```python
from build123d import *

# Parameters (mm, degrees)
SKETCH1_W                      = 58.7
SKETCH1_H                      = 85.15
SKETCH1_W_2                    = 230
SKETCH1_H_2                    = 50
BOSS_EXTRUDE1_DEPTH            = 10
M5_CLEARANCE_HOLE1_D           = 5.5
M5_CLEARANCE_HOLE1_CSINK_D     = 5.55
M5_CLEARANCE_HOLE1_CSINK_ANGLE = 90
SKETCH5_W                      = 40
SKETCH5_H                      = 50
CUT_EXTRUDE1_DEPTH             = 5
FILLET1_R                      = 10


# Read off the part's stored shape, not the designer's step: M5 Clearance Hole2
with BuildPart() as part:
    # Sketch1 → Boss-Extrude1 (new body)
    with BuildSketch(Plane(origin=(0, 0, 0), x_dir=(1, 0, 0), z_dir=(0, 1, 0))):
        with Locations((0, 67.575)):
            Rectangle(SKETCH1_W, SKETCH1_H)
        Rectangle(SKETCH1_W_2, SKETCH1_H_2)
    extrude(amount=BOSS_EXTRUDE1_DEPTH)

    # M5 Clearance Hole1 (through all)
    with Locations(Plane(origin=(0, 10, 0), x_dir=(1, 0, 0), z_dir=(0, 1, 0))):
        with Locations((-21.85, 52), (21.85, 52)):
            CounterSinkHole(M5_CLEARANCE_HOLE1_D / 2, M5_CLEARANCE_HOLE1_CSINK_D / 2, counter_sink_angle=M5_CLEARANCE_HOLE1_CSINK_ANGLE)

    # Sketch5 → Cut-Extrude1 (cut)
    with BuildSketch(Plane.XZ):
        with Locations((-95, 0)):
            Rectangle(SKETCH5_W, SKETCH5_H)
        with Locations((95, 0)):
            Rectangle(SKETCH5_W, SKETCH5_H)
    extrude(amount=-CUT_EXTRUDE1_DEPTH, mode=Mode.SUBTRACT)

    # M5 Clearance Hole2 outline → M5 Clearance Hole2 (revolve, cut)
    with BuildSketch(Plane(origin=(-85, 0, -15), x_dir=(1, 0, 0), z_dir=(0, 0, 1))):
        Polygon((2.75, 5.025), (2.75, 10), (0, 10), (0, 5), (2.775, 5), align=None)
    revolve(axis=Axis((-85, 0, -15), (0, 1, 0)), mode=Mode.SUBTRACT)

    # M5 Clearance Hole2 2 outline → M5 Clearance Hole2 2 (revolve, cut)
    with BuildSketch(Plane(origin=(-85, 0, 15), x_dir=(1, 0, 0), z_dir=(0, 0, 1))):
        Polygon((2.75, 5.025), (2.75, 10), (0, 10), (0, 5), (2.775, 5), align=None)
    revolve(axis=Axis((-85, 0, 15), (0, 1, 0)), mode=Mode.SUBTRACT)

    # M5 Clearance Hole2 3 outline → M5 Clearance Hole2 3 (revolve, cut)
    with BuildSketch(Plane(origin=(-105, 0, -15), x_dir=(1, 0, 0), z_dir=(0, 0, 1))):
        Polygon((2.75, 5.025), (2.75, 10), (0, 10), (0, 5), (2.775, 5), align=None)
    revolve(axis=Axis((-105, 0, -15), (0, 1, 0)), mode=Mode.SUBTRACT)

    # M5 Clearance Hole2 4 outline → M5 Clearance Hole2 4 (revolve, cut)
    with BuildSketch(Plane(origin=(-105, 0, 15), x_dir=(1, 0, 0), z_dir=(0, 0, 1))):
        Polygon((2.75, 5.025), (2.75, 10), (0, 10), (0, 5), (2.775, 5), align=None)
    revolve(axis=Axis((-105, 0, 15), (0, 1, 0)), mode=Mode.SUBTRACT)

    # M5 Clearance Hole2 5 outline → M5 Clearance Hole2 5 (revolve, cut)
    with BuildSketch(Plane(origin=(105, 0, -15), x_dir=(1, 0, 0), z_dir=(0, 0, 1))):
        Polygon((2.75, 5.025), (2.75, 10), (0, 10), (0, 5), (2.775, 5), align=None)
    revolve(axis=Axis((105, 0, -15), (0, 1, 0)), mode=Mode.SUBTRACT)

    # M5 Clearance Hole2 6 outline → M5 Clearance Hole2 6 (revolve, cut)
    with BuildSketch(Plane(origin=(105, 0, 15), x_dir=(1, 0, 0), z_dir=(0, 0, 1))):
        Polygon((2.75, 5.025), (2.75, 10), (0, 10), (0, 5), (2.775, 5), align=None)
    revolve(axis=Axis((105, 0, 15), (0, 1, 0)), mode=Mode.SUBTRACT)

    # M5 Clearance Hole2 7 outline → M5 Clearance Hole2 7 (revolve, cut)
    with BuildSketch(Plane(origin=(85, 0, -15), x_dir=(1, 0, 0), z_dir=(0, 0, 1))):
        Polygon((2.75, 5.025), (2.75, 10), (0, 10), (0, 5), (2.775, 5), align=None)
    revolve(axis=Axis((85, 0, -15), (0, 1, 0)), mode=Mode.SUBTRACT)

    # M5 Clearance Hole2 8 outline → M5 Clearance Hole2 8 (revolve, cut)
    with BuildSketch(Plane(origin=(85, 0, 15), x_dir=(1, 0, 0), z_dir=(0, 0, 1))):
        Polygon((2.75, 5.025), (2.75, 10), (0, 10), (0, 5), (2.775, 5), align=None)
    revolve(axis=Axis((85, 0, 15), (0, 1, 0)), mode=Mode.SUBTRACT)

    # Fillet1
    fillet1_edges = [part.edges().sort_by_distance(p)[0] for p in [
        (-29.35, 5, -110.15),
        (29.35, 5, -110.15),
        (29.35, 5, -25),
        (-29.35, 5, -25),
    ]]
    fillet(fillet1_edges, radius=FILLET1_R)


solid = part.part
```
Part model, mm, in its own coordinate system. A direction names the side the tool comes from. Give positions to 0.01 mm unless a question says otherwise; leave off trailing zeros. Loops run counter-clockwise (first coordinate to the right, second up) from the corner with the lowest first, then second, coordinate; pieces in that order, holes last. Notation, with made-up numbers: M 52,17 L 56,17 A24 ccw 56,48 Z; hole C -21,65 d6. An arc over 180 degrees is marked long. Return JSON: item names as keys, results as strings.
1) Saw through at A-A, the plane x = -85. List the corners of the cut face in (y, z) (3 decimals).
Calculated:
{"outline": "M 5,-25 L 10,-25 L 10,-17.75 L 5.025,-17.75 L 5,-17.775 Z; M 5,-12.225 L 5.025,-12.25 L 10,-12.25 L 10,12.25 L 5.025,12.25 L 5,12.225 Z; M 5,17.775 L 5.025,17.75 L 10,17.75 L 10,25 L 5,25 Z"}
2) Saw through at C-C, the plane x = 21.85. List the corners of the cut face in (y, z) (3 decimals), then the cut area to 3 significant figures.
Calculated:
{"outline": "M 0,-109.832 L 10,-109.832 L 10,-54.775 L 9.975,-54.75 L 0,-54.75 Z; M 0,-49.25 L 9.975,-49.25 L 10,-49.225 L 10,25 L 0,25 Z", "area": "1,290 mm2"}
3) Pull direction Z, two halves, no side cores. Call faces 1 (the face through (32.2, 5.07, -28.01)), 2 (the face through (-87.747, 7.547, -15.121)), 3 (the face through (95, 5, 0)): released by +Z, released by -Z, zero draft, split by the parting line, or undercut.
Calculated:
{"face 1": "released by -Z", "face 2": "undercut", "face 3": "zero draft"}
4) Drill centre lines: line 1 (Z direction, x = 105, y = 8.5); line 2 (X direction, y = 7.25, z = -15); line 3 (X direction, y = 6, z = -52). Where is each one in solid material? Low to high.
Calculated:
{"line 1": "z = -25 to -17.75, -12.25 to 12.25, 17.75 to 25", "line 2": "x = -115 to -107.75, -102.25 to -87.75, -82.25 to 82.25, 87.75 to 102.25, 107.75 to 115", "line 3": "x = -29.35 to -24.6, -19.1 to 19.1, 24.6 to 29.35"}
5) Flat gauge pins, fed straight in: pin 1 Ø9 at (x, z) = (-105, -15) entering from -Y; pin 2 Ø3 at (y, z) = (2.5, -85.5) entering from -X; pin 3 Ø5.5 at (y, z) = (3, 3.5) entering from +X; pin 4 Ø3 at (y, z) = (5.5, -42.5) entering from +X. Where does each tip first touch, or does it go through?
Calculated:
{"pin 1": "stops at y = 5", "pin 2": "stops at x = -29.35", "pin 3": "stops at x = 115", "pin 4": "stops at x = 29.35"}
6) 3-axis set-ups, long thin cutter, end or side, ignore diameter. For faces 4 (the face through (-69, 6, -25)), 5 (the face through (29.35, 5, -67)), 6 (the face through (115, 7, 0)): which of +Z, -Z, +X, -X, +Y, -Y reach the whole face in a straight line?
Calculated:
{"face 4": "-Z, -X, +Y, -Y", "face 5": "-Z, +X, +Y, -Y", "face 6": "+Z, -Z, +X, +Y, -Y"}
7) Saw through at B-B, the plane y = 7.25. Count the separate pieces of the cut face and the enclosed holes in it, then the cut area to 3 significant figures.
Calculated:
{"separate pieces": "1", "enclosed holes": "10", "area": "16,300 mm2"}
8) Saw through at D-D, the plane x = 52.5. List the corners of the cut face in (y, z).
Calculated:
{"outline": "M 0,-25 L 10,-25 L 10,25 L 0,25 Z"}
